For this review, take the finished solid that the model builds, in its own axes (mm). Round coordinates to 2 decimals unless told otherwise and drop trailing zeros. Write each loop counter-clockwise with the first axis right and the second up, starting at its lowest first coordinate (ties: lowest second). Pieces come first, ordered by that corner, then holes. Notation, with made-up numbers: (-11, 37) -> (39, 37) arc R17 ccw to (39, 42) -> close; hole circle Ø2 at (19.5, 13.5). An arc over 180 degrees is marked (long way). Answer in a Markdown table with one row per item. Add a question column.
```python
from build123d import *

# Parameters (mm, degrees)
F1_DEPTH = 6
F3_D     = 4.1
F4_D     = 8
F5_D     = 7.8
F6_R     = 15


with BuildPart() as f1:
    # F0 (on Front) → F1 (new body)
    with BuildSketch(Plane.XZ):
        with BuildLine():
            Line((7.4858944747, 0.4597650633), (5.9971782314, 48.9839925561))
            ThreePointArc((5.9971782314, 48.9839925561), (-0.0920070963, 54.7992945164), (-6, 48.8))
            Line((-6, 48.8), (-7.2834242523, 7.1447653329))
            Line((-7.2834242523, 7.1447653329), (-30.3, 5.9924953066))
            ThreePointArc((-30.3, 5.9924953066), (-35.9999999283, -0.0009276797), (-30.298146947, -5.9925877881))
            Line((-30.298146947, -5.9925877881), (-0.7444465641, -7.4629618325))
            Line((-0.7444465641, -7.4629618325), (0, -7.5))
            ThreePointArc((0, -7.5), (5.3033008589, -5.3033008589), (7.5, 0))
            Line((7.5, 0), (7.4858944747, 0.4597650633))
        make_face()
    extrude(amount=-F1_DEPTH)

    # F3 (through all)
    with Locations(Plane.XZ):
        with Locations((-30, 0)):
            Hole(F3_D / 2)

    # F4 (through all)
    with Locations(Plane.XZ):
        with Locations((0, 48.8)):
            Hole(F4_D / 2)

    # F5 (through all)
    with Locations(Plane.XZ):
        with Locations((0, 0)):
            Hole(F5_D / 2)

    # F6
    f6_edges = [f1.edges().sort_by_distance(p)[0] for p in [
        (-7.283424, 3, 7.144765),
    ]]
    fillet(f6_edges, radius=F6_R)


solid = f1.part
```
1. For L1, parallel to Z at x = 0, y = 3.7; L2, parallel to Z at x = 3.5, y = 5.1; L3, parallel to Z at x = -30, y = 4.35, list the stretches that pass through material, from the lowest coordinate up. Write a range as [from, to].
2. We need section C-C (x = -24.5). Write out the cut boundary in (y, z), plus the area to 3 significant figures.
3. We need section B-B (z = 3). Write out the cut boundary in (x, y).
4. The part is to be moulded in two halves that separate along X. For faces 1 (the flat face through (-5, 6, 17)), 2 (the cylindrical face through (-36, 3, 0)), 3 (the cylindrical face through (0, 3, 54.8)), 4 (the cylindrical face through (0.521, 3.042, 52.766)), say which applies: pulls with the +X half, pulls with the -X half, needs draft (parallel to the pull), parting line crosses it, or undercut.
5. We need section D-D (z = 15.5). Write out the cut boundary in (x, y).
6. We need section A-A (y = 3.8). Write out the cut boundary in (x, z).
7. Clearance check with flat-ended pins moving along their axes: pin 1 Ø10 at (x, z) = (-13, 10) entering from +Y; pin 2 Ø2 at (x, y) = (-14, 3) entering from -Z; pin 3 Ø3 at (x, y) = (-11.5, 5) entering from -Z; pin 4 Ø1.5 at (x, y) = (-26, 1) entering from -Z. State where each tip first meets the part, or that it passes through.
Response:
| question | item | result |
|---|---|---|
| 1 | L1 | [-7.5, -3.9], [3.9, 44.8], [52.8, 54.8] |
| 1 | L2 | [-6.63, -1.72], [1.72, 46.86], [50.74, 53.67] |
| 1 | L3 | [-6.01, -2.05], [2.05, 6.01] |
| 2 | outline | (0, -6.28) -> (6, -6.28) -> (6, 6.28) -> (0, 6.28) -> close |
| 2 | area | 75.4 mm2 |
| 3 | outline | (-35.2, 0) -> (-2.49, 0) -> (-2.49, 6) -> (-35.2, 6) -> close; (2.49, 0) -> (7.41, 0) -> (7.41, 6) -> (2.49, 6) -> close |
| 4 | face 1 | needs draft |
| 4 | face 2 | pulls with the -X half |
| 4 | face 3 | parting line crosses it |
| 4 | face 4 | undercut |
| 5 | outline | (-8.07, 0) -> (7.02, 0) -> (7.02, 6) -> (-8.07, 6) -> close |
| 6 | outline | (-30.3, -5.99) -> (0, -7.5) arc R7.5 ccw to (7.5, 0) -> (6, 48.98) arc R6 ccw to (-6, 48.8) -> (-6.86, 20.97) arc R15 cw to (-21.1, 6.45) -> (-30.3, 5.99) arc R6 ccw to start; hole circle Ø4.1 at (-30, 0); hole circle Ø8 at (0, 48.8); hole circle Ø7.8 at (0, 0) |
| 7 | pin 1 | y = 6 |
| 7 | pin 2 | z = -6.85 |
| 7 | pin 3 | z = -7 |
| 7 | pin 4 | z = -6.24 |
